```python
from build123d import *

# Parameters (mm, degrees)
SKETCH1_R           = 3
BOSS_EXTRUDE1_DEPTH = 3.175


with BuildPart() as part:
    # Sketch1 → Boss-Extrude1 (new body)
    with BuildSketch(Plane.XY):
        with BuildLine():
            Line((25, 170), (175, 170))
            ThreePointArc((175, 170), (223.684930832, 189.383563894), (275, 200))
            Line((275, 200), (278.48892965, 170.203567833))
            ThreePointArc((278.48892965, 170.203567833), (228.984362684, 159.629140364), (182.323699215, 140))
            Line((182.323699215, 140), (17.676300785, 140))
            ThreePointArc((17.676300785, 140), (-27.163176857, 159.050053662), (-74.696057289, 169.732215313))
            add(Edge.make_bspline(
                [(-459.597813184, -125.74437106), (-458.167847661, -124.888859924), (-455.300989911, -123.160410804), (-449.693031194, -119.725805066), (-442.844497858, -115.430194443), (-434.897527213, -110.280573748), (-424.643042919, -103.410605598), (-412.446207366, -94.807407336), (-398.73286692, -84.425459971), (-385.875530014, -73.956655832), (-369.787206696, -59.850046206), (-355.152571956, -45.476802835), (-341.718077927, -30.784744771), (-332.160906415, -19.581186548), (-323.101555816, -8.241034683), (-311.630816912, 6.863649777), (-298.117522758, 25.605990916), (-282.395742384, 47.431562205), (-266.384320483, 68.25099024), (-249.34123977, 87.803395961), (-230.504956306, 105.928130356), (-212.601243201, 119.774018212), (-196.457396921, 130.048920131), (-183.303935629, 137.33205425), (-168.969219752, 144.162376514), (-153.317967868, 150.50005901), (-136.218766867, 156.296597686), (-120.658812709, 160.629761276), (-107.364076993, 163.767973943), (-96.958515184, 165.949209965), (-87.903435435, 167.618170459), (-80.445251901, 168.856738216), (-76.604810273, 169.448930821), (-74.696057289, 169.732215313)],
                knots=[0, 0, 0, 0, 0.007772041, 0.015544083, 0.031088165, 0.046632248, 0.06217633, 0.093264496, 0.124352661, 0.155440826, 0.186528991, 0.248705321, 0.279793487, 0.310881652, 0.341969817, 0.373057982, 0.435234312, 0.497410643, 0.559586973, 0.621763303, 0.683939634, 0.746115964, 0.777204129, 0.808292294, 0.83938046, 0.870468625, 0.90155679, 0.932644955, 0.948189038, 0.96373312, 0.979277203, 0.987049244, 0.994821285, 0.994821285, 0.994821285, 0.994821285], degree=3))
            Line((-459.597813184, -125.74437106), (-494.597813184, -200.74437106))
            Line((-494.597813184, -200.74437106), (-554.962766018, -200.74437106))
            Line((-554.962766018, -200.74437106), (-554.962766018, -125.74437106))
            Line((-554.962766018, -125.74437106), (-534.962766018, -125.74437106))
            Line((-534.962766018, -125.74437106), (-534.962766018, -180.74437106))
            Line((-534.962766018, -180.74437106), (-519.962766018, -180.74437106))
            Line((-519.962766018, -180.74437106), (-475, -100))
            add(Edge.make_bspline(
                [(-475, -100), (-419.540575809, -66.820070684), (-306.013905785, 34.036801702), (-257.635554762, 174.287094016), (-75, 200)],
                knots=[0, 0, 0, 0, 0.312223899, 1, 1, 1, 1], degree=3))
            ThreePointArc((-75, 200), (-23.684930832, 189.383563894), (25, 170))
        make_face()
        with Locations((-412.174499428, -75.74437106)):
            Circle(SKETCH1_R, mode=Mode.SUBTRACT)
        with Locations((-317.601811803, 24.25562894)):
            Circle(SKETCH1_R, mode=Mode.SUBTRACT)
        with Locations((-231.096695012, 124.25562894)):
            Circle(SKETCH1_R, mode=Mode.SUBTRACT)
        with Locations((-127.411512689, 174.25562894)):
            Circle(SKETCH1_R, mode=Mode.SUBTRACT)
        with Locations((100, 155)):
            Circle(SKETCH1_R, mode=Mode.SUBTRACT)
        with Locations((226.311251147, 174.505328628)):
            Circle(SKETCH1_R, mode=Mode.SUBTRACT)
        with Locations((-25.392583218, 174.221837866)):
            Circle(SKETCH1_R, mode=Mode.SUBTRACT)
    extrude(amount=BOSS_EXTRUDE1_DEPTH)


solid = part.part
```
The listing builds one solid part. Answer for the finished solid, in the listing's coordinates (mm). A direction names the side the tool comes from. Coordinates: 2 decimals unless noted, no trailing zeros. Loops run counter-clockwise (first coordinate to the right, second up) from the corner with the lowest first, then second, coordinate; pieces in that order, holes last. Notation, with made-up numbers: (62.25, 63) - (85.25, 63) arc R16 ccw to (85.25, 89) - close; hole circle Ø3 at (86.25, 42). An arc over 180 degrees is marked (long way). Write item = value, one per line.
1) Section C-C (z = 2.15) is taken. Count the separate pieces of the cut face and the enclosed holes in it, plus the area to 3 significant figures.
Responses:
separate_pieces = 1
enclosed_holes = 7
area = 30,400 mm^2
2) Section B-B (x = 141.5) is taken. Determine the outline of the cut face in (y, z) (3 decimals).
Responses:
outline = (140, 0) - (170, 0) - (170, 3.175) - (140, 3.175) - close
3) Section A-A (y = -158) is taken. Determine the outline of the cut face in (x, z) (3 decimals), plus the area to 3 significant figures.
Responses:
outline = (-554.963, 0) - (-534.963, 0) - (-534.963, 3.175) - (-554.963, 3.175) - close; (-507.297, 0) - (-474.65, 0) - (-474.65, 3.175) - (-507.297, 3.175) - close
area = 167 mm^2
4) Which of the six approach directions +Z, -Z, +X, -X, +Y, -Y give full straight-line access (tool end or side, diameter ignored) to faces 1 (the face through (222.98, 189.17, 1.57)), 2 (the face through (-26.51, 158.84, 1.57)), 3 (the face through (-476.853, -162.719, 1.565))?
Responses:
face_1 = +Z, -Z, +Y
face_2 = +Z, -Z, -Y
face_3 = +Z, -Z, +X, -Y
5) Determine the mould class of faces 4 (the face through (-497.796, -140.937, 1.565)), 5 (the face through (-24.389, 189.594, 1.565)), 6 (the face through (229.66, 159.84, 1.57)), 7 (the face through (-198, 134, 3.175)) for opening direction X: pulls with the +X half, pulls with the -X half, needs draft (parallel to the pull), parting line crosses it, or undercut.
Responses:
face_4 = undercut
face_5 = undercut
face_6 = pulls with the +X half
face_7 = needs draft
6) Find the intervals of material crossed by line 1 along X through (y, z) = (172, 0.65); line 2 along X through (y, z) = (141.5, 2.2); line 3 along X through (y, z) = (-177, 1.3), in increasing order.
Responses:
line_1 = -179.78 to -129.39, -125.43 to -27.41, -23.38 to 20.95, 179.05 to 224.66, 227.96 to 278.28
line_2 = -233.19 to -174.45, 14.84 to 185.16
line_3 = -554.96 to -534.96, -517.88 to -483.52
7) Each of these flat-tipped pins is pushed along its axis until it touches: P1, Ø1.6, axis at x = -545.5, z = 1, coming from the +Y side; P2, Ø1, axis at x = -526.5, z = 2, coming from the +Y side; P3, Ø1.6, axis at y = -164.5, z = 2, coming from the +X side. Where does it stop, or does it pass through?
Responses:
P1 = -125.74
P2 = -180.74
P3 = -477.31
